Part model, mm, in its own coordinate system. Face numbers are marked on the shaded views. A direction names the side the tool comes from. Give positions to 0.01 mm unless a question says otherwise; leave off trailing zeros. Write each loop counter-clockwise with the first axis right and the second up, starting at its lowest first coordinate (ties: lowest second). Pieces come first, ordered by that corner, then holes.
from build123d import *

# Parameters (mm, degrees)
SKETCH1_R           = 6
BOSS_EXTRUDE1_DEPTH = 10
SKETCH2_R           = 12
BOSS_EXTRUDE2_DEPTH = 4
SKETCH3_R           = 8
BOSS_EXTRUDE3_DEPTH = 41
SKETCH4_R           = 6
BOSS_EXTRUDE4_DEPTH = 6
CHAMFER1_SIZE       = 1
CHAMFER2_SIZE       = 1
CHAMFER3_SIZE       = 1
CUT_EXTRUDE1_DEPTH  = 1.8


with BuildPart() as part:
    # Sketch1 → Boss-Extrude1 (new body)
    with BuildSketch(Plane(origin=(0, 0, 0), x_dir=(1, 0, 0), z_dir=(0, 1, 0))):
        with Locations(Location((0, 0, 0), (0, 0, 270))):
            Circle(SKETCH1_R)
    extrude(amount=BOSS_EXTRUDE1_DEPTH)

    # Sketch2 → Boss-Extrude2 (add)
    with BuildSketch(Plane(origin=(0, 10, 0), x_dir=(1, 0, 0), z_dir=(0, 1, 0))):
        with Locations(Location((0, 0, 0), (0, 0, 270))):
            Circle(SKETCH2_R)
    extrude(amount=BOSS_EXTRUDE2_DEPTH)

    # Sketch3 → Boss-Extrude3 (add)
    with BuildSketch(Plane(origin=(0, 14, 0), x_dir=(1, 0, 0), z_dir=(0, 1, 0))):
        with Locations(Location((0, 0, 0), (0, 0, 270))):
            Circle(SKETCH3_R)
    extrude(amount=BOSS_EXTRUDE3_DEPTH)

    # Sketch4 → Boss-Extrude4 (add)
    with BuildSketch(Plane(origin=(0, 55, 0), x_dir=(1, 0, 0), z_dir=(0, 1, 0))):
        with Locations(Location((0, 0, 0), (0, 0, 270))):
            Circle(SKETCH4_R)
    extrude(amount=BOSS_EXTRUDE4_DEPTH)

    # Chamfer1
    chamfer1_edges = [part.edges().sort_by_distance(p)[0] for p in [
        (0, 0, -6),
    ]]
    chamfer(chamfer1_edges, length=CHAMFER1_SIZE)

    # Chamfer2
    chamfer2_edges = [part.edges().sort_by_distance(p)[0] for p in [
        (0, 61, -6),
    ]]
    chamfer(chamfer2_edges, length=CHAMFER2_SIZE)

    # Chamfer3
    chamfer3_edges = [part.edges().sort_by_distance(p)[0] for p in [
        (0, 55, -8),
    ]]
    chamfer(chamfer3_edges, length=CHAMFER3_SIZE)

    # Sketch5 → Cut-Extrude1 (cut)
    with BuildSketch(Plane(origin=(8, 0, 0), x_dir=(0, 0, -1), z_dir=(1, 0, 0))):
        with BuildLine():
            Line((2.5, 42.5), (2.5, 27.5))
            ThreePointArc((2.5, 27.5), (0, 25), (-2.5, 27.5))
            Line((-2.5, 27.5), (-2.5, 42.5))
            ThreePointArc((-2.5, 42.5), (0, 45), (2.5, 42.5))
        make_face()
    extrude(amount=-CUT_EXTRUDE1_DEPTH, mode=Mode.SUBTRACT)


solid = part.part
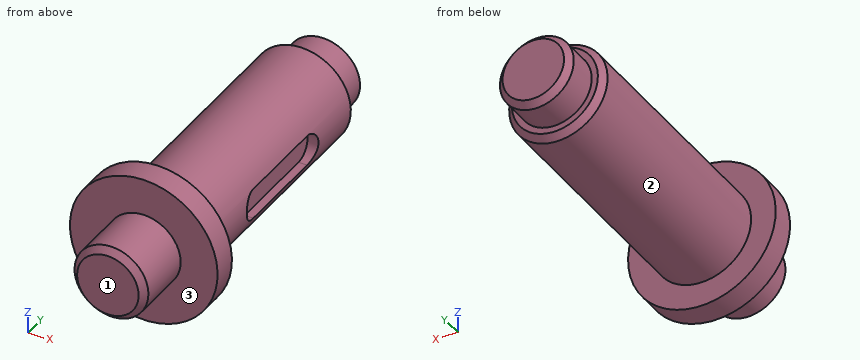
1) Saw through at A-A (x = 9.5). Write the cut outline in (y, z).
Check result:
outline: (10, -7.33) - (14, -7.33) - (14, 7.33) - (10, 7.33) - close
2) Flat gauge pins, fed straight in: P1, Ø8, axis at x = 9, y = 33.5, coming from the +Z side (3 decimals); P2, Ø4, axis at y = 7.5, z = 7, coming from the -X side; P3, Ø8, axis at x = 7, y = 21.5, coming from the +Z side. Where does each tip first touch, or does it go through?
Check result:
P1: stops at z = 6.245
P2: stops at x = -3.32
P3: stops at z = 7.42
3) Drill centre lines: L1, parallel to Y at x = -9.25, z = 6.75; L2, parallel to Y at x = 7, z = -2; L3, parallel to X at y = 7.5, z = -0.25. Where is each one in solid material? Low to high.
Check result:
L1: y = 10 to 14
L2: y = 10 to 26, 44 to 54.72
L3: x = -5.99 to 5.99
4) 3-axis set-ups, long thin cutter, end or side, ignore diameter. For the marked faces 1, 2 and 3: which of +Z, -Z, +X, -X, +Y, -Y reach the whole face in a straight line?
Check result:
face 1: +Z, -Z, +X, -X, -Y
face 2: +Y
face 3: -Y
